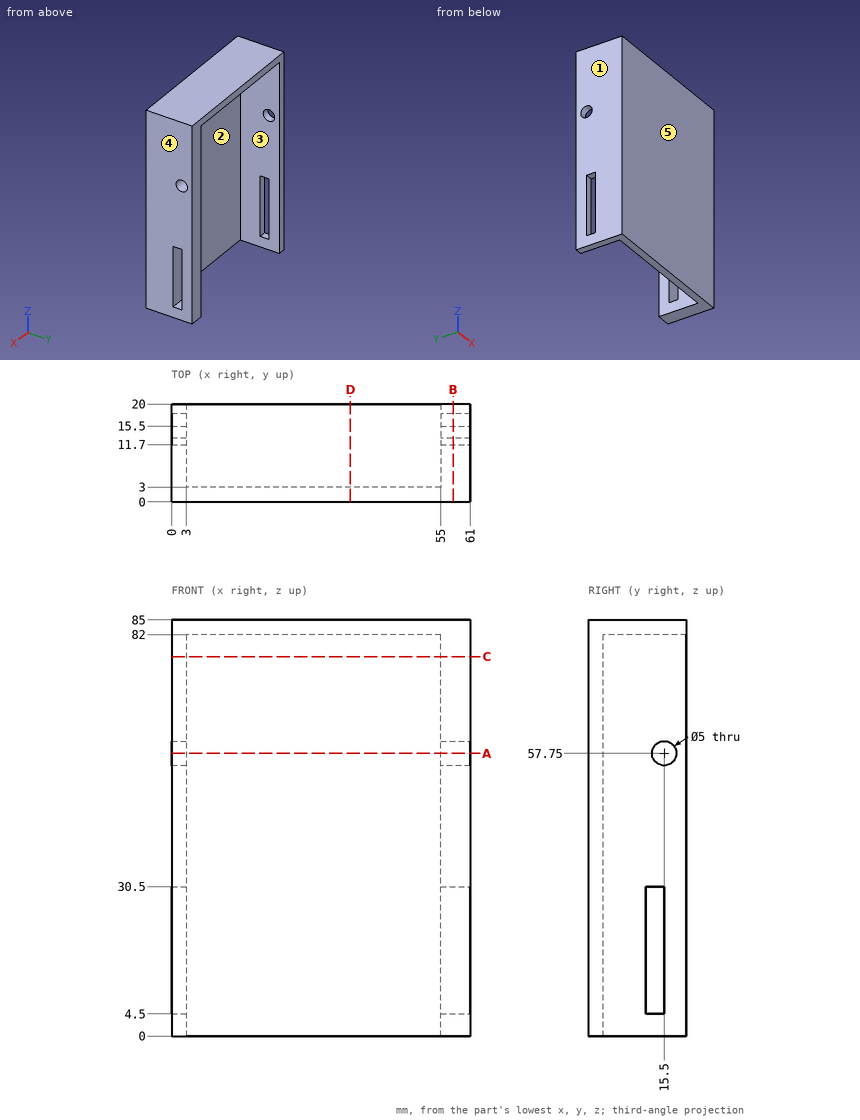
The figure shows three views and two pictorial views of one solid part (mm, origin at its lowest corner). Answer the questions. A direction names the side the tool comes from. Coordinates: 2 decimals unless noted, no trailing zeros. Write each loop counter-clockwise with the first axis right and the second up, starting at its lowest first coordinate (ties: lowest second). Pieces come first, ordered by that corner, then holes. Notation, with made-up numbers: (10.5, -7) -> (60.5, -7) arc R12 cw to (60.5, 13) -> close; hole circle Ø11 at (12.5, 45.25). An arc over 180 degrees is marked (long way). Return JSON: item names as keys, results as strings.
(1) For a pull along X with two mould halves and no side action, classify the marked faces 3, 4 and 5 as pulls with the +X half, pulls with the -X half, needs draft (parallel to the pull), parting line crosses it, or undercut.
Answers below:
{"face 3": "undercut", "face 4": "pulls with the +X half", "face 5": "needs draft"}
(2) Consider line 1 along X through (y, z) = (9, 77); line 2 along Y through (x, z) = (1.25, 57.75); line 3 along Z through (x, y) = (32, 17). Determine where each line is inside the solid, lowest interval first. Write a range as from..to.
Answers below:
{"line 1": "0..3, 55..61", "line 2": "0..13, 18..20", "line 3": "82..85"}
(3) Each of these flat-tipped pins is pushed along its axis until it touches: P1, Ø1, axis at x = 28, y = 5, coming from the -Z side; P2, Ø2, axis at x = 40, z = 12, coming from the +Y side. Where does it stop, or does it pass through?
Answers below:
{"P1": "z = 82", "P2": "y = 3"}
(4) The part is cut by section A-A on z = 57.75. Give the vertices of the cut face in (x, y).
Answers below:
{"outline": "(0, 0) -> (61, 0) -> (61, 13) -> (55, 13) -> (55, 3) -> (3, 3) -> (3, 13) -> (0, 13) -> close; (0, 18) -> (3, 18) -> (3, 20) -> (0, 20) -> close; (55, 18) -> (61, 18) -> (61, 20) -> (55, 20) -> close"}
(5) The part is cut by section D-D on x = 36.5. Give the vertices of the cut face in (y, z), then the cut area to 3 significant figures.
Answers below:
{"outline": "(0, 0) -> (3, 0) -> (3, 82) -> (20, 82) -> (20, 85) -> (0, 85) -> close", "area": "306 mm^2"}
(6) The part is cut by section C-C on z = 77.5. Give the vertices of the cut face in (x, y), then the cut area to 3 significant figures.
Answers below:
{"outline": "(0, 0) -> (61, 0) -> (61, 20) -> (55, 20) -> (55, 3) -> (3, 3) -> (3, 20) -> (0, 20) -> close", "area": "336 mm^2"}
(7) The part is cut by section B-B on x = 57.5. Give the vertices of the cut face in (y, z), then the cut area to 3 significant figures.
Answers below:
{"outline": "(0, 0) -> (20, 0) -> (20, 85) -> (0, 85) -> close; hole (11.7, 4.5) -> (15.5, 4.5) -> (15.5, 30.5) -> (11.7, 30.5) -> close; hole circle Ø5 at (15.5, 57.75)", "area": "1,580 mm^2"}
(8) Which of the six approach directions +Z, -Z, +X, -X, +Y, -Y give full straight-line access (tool end or side, diameter ignored) to the marked faces 1 and 2?
Answers below:
{"face 1": "+Z, -Z, -X, +Y, -Y", "face 2": "-Z, +Y"}
